Build history of the part. All positions in model axes, mm. Give positions to 0.01 mm unless a question says otherwise; leave off trailing zeros. Loops run counter-clockwise (first coordinate to the right, second up) from the corner with the lowest first, then second, coordinate; pieces in that order, holes last. Notation, with made-up numbers: M 38.25,-11 L 58.25,-11 A31 ccw 58.25,18 Z; hole C 28.25,-37 d9. An arc over 180 degrees is marked long. Answer as a JSON object with one key per item and string values. Group by question number.
1. Drill centre lines: line 1 along Z through (x, y) = (-15, -10); line 2 along X through (y, z) = (-5.5, 0). Where is each one in solid material? Low to high. Write a range as [from, to].
2. Drop flat-ended pins along their axis: pin 1 Ø10 at (x, z) = (-15, 15) entering from +Y; pin 2 Ø7.5 at (x, z) = (-15, -15) entering from +Y. Give the stop position or say it passes through.
3. Mould opens along X. For faces 1 (the face through (11.876, -7.967, 15.694)), 2 (the face through (-0.3, 0, -11.5)), 3 (the face through (24.14, -6.44, -24.1)), 4 (the face through (-17.04, -2.95, -12.34)) say: released by +X, released by -X, zero draft, split by the parting line, or undercut.
4. Slice it at C-C (x = -15). List the corners of the cut face in (y, z), then the cut area to 3 significant figures.
5. Slice it at A-A (z = -15). List the corners of the cut face in (x, y), then the cut area to 3 significant figures.
6. Slice it at B-B (y = -11). List the corners of the cut face in (x, z), then the cut area to 3 significant figures.
7. Slice it at D-D (x = 0). List the corners of the cut face in (y, z).
from build123d import *

# Parameters (mm, degrees)
SKETCH2_W                                       = 50
SKETCH2_H                                       = 50
SKETCH2_R                                       = 10.993
BOSS_EXTRUDE1_DEPTH                             = 12.7
CSK_FOR_M6_FLAT_HEAD_MACHINE_SCREW1_D           = 6.4
CSK_FOR_M6_FLAT_HEAD_MACHINE_SCREW1_CSINK_D     = 12.6
CSK_FOR_M6_FLAT_HEAD_MACHINE_SCREW1_CSINK_ANGLE = 90
FILLET1_R                                       = 3


with BuildPart() as part:
    # Sketch2 → Boss-Extrude1 (new body)
    with BuildSketch(Plane(origin=(0, 0, 0), x_dir=(1, 0, 0), z_dir=(0, 1, 0))):
        Rectangle(SKETCH2_W, SKETCH2_H)
        with Locations(Location((0, 0, 0), (0, 0, 270))):
            Circle(SKETCH2_R, mode=Mode.SUBTRACT)
    extrude(amount=-BOSS_EXTRUDE1_DEPTH)

    # CSK for M6 Flat Head Machine Screw1 (through all)
    with Locations(Plane(origin=(-15, 0, 15), x_dir=(0, 0, 1), z_dir=(0, 1, 0))):
        with Locations((0, 0), (0, 30), (-30, 0), (-30, 30)):
            CounterSinkHole(CSK_FOR_M6_FLAT_HEAD_MACHINE_SCREW1_D / 2, CSK_FOR_M6_FLAT_HEAD_MACHINE_SCREW1_CSINK_D / 2, counter_sink_angle=CSK_FOR_M6_FLAT_HEAD_MACHINE_SCREW1_CSINK_ANGLE)

    # Fillet1
    fillet1_edges = [part.edges().sort_by_distance(p)[0] for p in [
        (-25, -6.35, -25),
        (25, -6.35, -25),
        (25, -6.35, 25),
        (-25, -6.35, 25),
    ]]
    fillet(fillet1_edges, radius=FILLET1_R)


solid = part.part
Established:
{
 "1": {"line 1": "z = [-25, -18.2], [-11.8, 11.8], [18.2, 25]", "line 2": "x = [-25, -10.99], [10.99, 25]"},
 "2": {"pin 1": "stops at y = -1.3", "pin 2": "stops at y = -2.55"},
 "3": {"face 1": "undercut", "face 2": "zero draft", "face 3": "released by +X", "face 4": "undercut"},
 "4": {"outline": "M -12.7,-25 L 0,-25 L 0,-21.3 L -3.1,-18.2 L -12.7,-18.2 Z; M -12.7,-11.8 L -3.1,-11.8 L 0,-8.7 L 0,8.7 L -3.1,11.8 L -12.7,11.8 Z; M -12.7,18.2 L -3.1,18.2 L 0,21.3 L 0,25 L -12.7,25 Z", "area": "453 mm^2"},
 "5": {"outline": "M -25,-12.7 L -18.2,-12.7 L -18.2,-3.1 L -21.3,0 L -25,0 Z; M -11.8,-12.7 L 11.8,-12.7 L 11.8,-3.1 L 8.7,0 L -8.7,0 L -11.8,-3.1 Z; M 18.2,-12.7 L 25,-12.7 L 25,0 L 21.3,0 L 18.2,-3.1 Z", "area": "453 mm^2"},
 "6": {"outline": "M -25,-22 A3 ccw -22,-25 L 22,-25 A3 ccw 25,-22 L 25,22 A3 ccw 22,25 L -22,25 A3 ccw -25,22 Z; hole C -15,-15 d6.4; hole C -15,15 d6.4; hole C 0,0 d21.99; hole C 15,-15 d6.4; hole C 15,15 d6.4", "area": "1,980 mm^2"},
 "7": {"outline": "M -12.7,-25 L 0,-25 L 0,-10.99 L -12.7,-10.99 Z; M -12.7,10.99 L 0,10.99 L 0,25 L -12.7,25 Z"}
}
